Model file for the job. Use its own axes, mm. Face numbers are marked on the shaded views. Round coordinates to 2 decimals unless told otherwise and drop trailing zeros. Loops run counter-clockwise (first coordinate to the right, second up) from the corner with the lowest first, then second, coordinate; pieces in that order, holes last. Notation, with made-up numbers: M 68,14 L 120,14 A17 ccw 120,34 Z; hole C -4,5 d6. An arc over 180 degrees is marked long. Use a Markdown table: item, result. Add a question column.
Q1. Pin check, flat tip, straight feed: pin 1 (2.5 mm diameter, centred on x = -20, y = 5, fed in from -Z). Stop position of the tip, or through.
Q2. Mould opens along Z. For the marked faces 1, 2, 3 and 4 say: +Z half, -Z half, draft (parallel to the pull), parting line (faces both ways), or undercut.
Q3. Cut at D-D (x = -60). Give the cut face in (y, z), plus the area to 3 significant figures.
Q4. Cut at B-B (x = -37). Give the cut face in (y, z).
Q5. Cut at A-A (y = 5). Give the cut face in (x, z), plus the area to 3 significant figures.
Q6. Cut at C-C (z = 6.35). Give the cut face in (x, y), plus the area to 3 significant figures.
Q7. Probe line 1 (Y direction, x = -75, z = 6); line 2 (Z direction, x = -43, y = 2.5); line 3 (X direction, y = 5, z = 9.25). List the from-to ranges inside material, lowest first. Write a range as from..to.
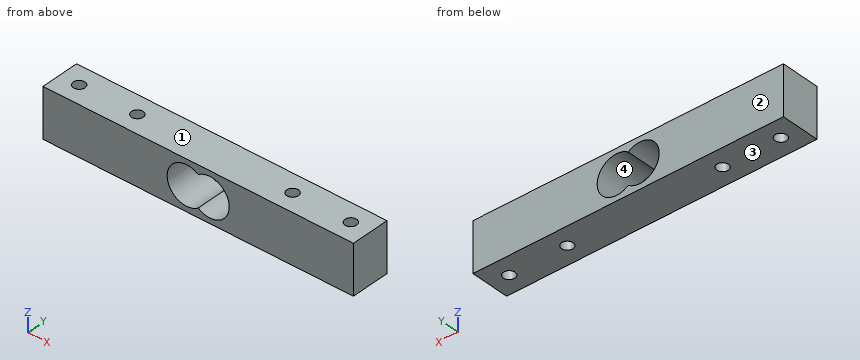
Autodesk Inventor part; units mm, degrees
ref_plane "YZ Plane" through (0, 0, 0) normal (1, 0, 0) x (0, 1, 0)
ref_plane "XZ Plane" through (0, 0, 0) normal (0, 1, 0) x (-1, 0, 0)
ref_plane "XY Plane" through (0, 0, 0) normal (0, 0, 1) x (1, 0, 0)
sketch "Sketch1" plane through (0, 0, 0) normal (0, 0, 1) x (1, 0, 0)
  line L0 (-80, 10) -> (0, 10)
  line L1 (0, 10) -> (0, 0)
  line L2 (0, 0) -> (-80, 0)
  line L3 (-80, 0) -> (-80, 10)
  line L4 (-40, 0) -> (-40, 10) construction
  line L5 (-80, 5) -> (0, 5) construction
  point P0 (-75, 5)
  point P1 (-60, 5)
  point P2 (-5, 5)
  point P3 (-20, 5)
  dimension "load_cell_length" = 80
  dimension "load_cell_width" = 10
  dimension "load_cell_hole_inset" = 5
  dimension "load_cell_hole_spacing" = 15
extrude "Extrusion1" add sketch "Sketch1" along normal blind 12.7
hole "Hole1" at (-5, 5, 0) at (-20, 5, 0) at (-60, 5, 0) at (-75, 5, 0) direction (0, 0, 1) diameter 3 end through all
thread "Thread1"
thread "Thread2"
thread "Thread3"
thread "Thread4"
sketch "Sketch3" plane through (-80, 10, 0) normal (0, 1, 0) x (1, 0, 0)
  line L0 (80, 0) -> (0, 0) construction
  line L1 (0, 0) -> (0, -12.7) construction
  line L2 (80, -12.7) -> (0, -12.7) construction
  line L3 (80, 0) -> (80, -12.7) construction
  line L4 (0, -6.35) -> (80, -6.35)
  line L5 (40, -12.7) -> (40, 0)
  arc A0 (40, -2.35) -> (40, -10.35) centre (37, -6.35) ccw
  arc A1 (40, -10.35) -> (40, -2.35) centre (43, -6.35) ccw
  dimension "d23" = 10
  dimension "d24" = 6
extrude "Extrusion3" cut sketch "Sketch3" against normal blind 10
equation "\"d25\" = d23"
properties part number "load_cell"
Checked values:
| question | item | result |
|---|---|---|
| 1 | pin 1 | passes through |
| 2 | face 1 | +Z half |
| 2 | face 2 | draft |
| 2 | face 3 | -Z half |
| 2 | face 4 | undercut |
| 3 | outline | M 0,0 L 3.5,0 L 3.5,12.7 L 0,12.7 Z; M 6.5,0 L 10,0 L 10,12.7 L 6.5,12.7 Z |
| 3 | area | 88.9 mm^2 |
| 4 | outline | M 0,0 L 10,0 L 10,1.35 L 0,1.35 Z; M 0,11.35 L 10,11.35 L 10,12.7 L 0,12.7 Z |
| 5 | outline | M -80,0 L -76.5,0 L -76.5,12.7 L -80,12.7 Z; M -73.5,0 L -61.5,0 L -61.5,12.7 L -73.5,12.7 Z; M -58.5,0 L -21.5,0 L -21.5,12.7 L -58.5,12.7 Z; M -18.5,0 L -6.5,0 L -6.5,12.7 L -18.5,12.7 Z; M -3.5,0 L 0,0 L 0,12.7 L -3.5,12.7 Z; hole M -40,2.35 A5 ccw long -40,10.35 A5 ccw long Z |
| 5 | area | 729 mm^2 |
| 6 | outline | M -80,0 L -48,0 L -48,10 L -80,10 Z; M -32,0 L 0,0 L 0,10 L -32,10 Z; hole C -75,5 d3; hole C -60,5 d3; hole C -20,5 d3; hole C -5,5 d3 |
| 6 | area | 612 mm^2 |
| 7 | line 1 | y = 0..3.5, 6.5..10 |
| 7 | line 2 | z = 0..1.35, 11.35..12.7 |
| 7 | line 3 | x = -80..-76.5, -73.5..-61.5, -58.5..-47.07, -32.93..-21.5, -18.5..-6.5, -3.5..0 |
